Geometry: final body of the model. Coordinates: model frame, mm. A direction names the side the tool comes from. Round coordinates to 2 decimals unless told otherwise and drop trailing zeros. Loops run counter-clockwise (first coordinate to the right, second up) from the corner with the lowest first, then second, coordinate; pieces in that order, holes last. Notation, with made-up numbers: (-29.5, -0.75) - (-8.5, -0.75) arc R17 ccw to (-8.5, 11.25) - close; hole circle Ø11 at (15, 38.5). An arc over 180 degrees is marked (long way). Write item = value, one per line. Start each with the question number.
Item 1: Section B-B (y = 7.75). Return loops of the section in (x, z), plus the area to 3 significant figures.
Item 2: Line query: line 1 (Z direction, x = -1.75, y = 3); line 2 (X direction, y = 3.75, z = 3.5); line 3 (X direction, y = 5.25, z = 48). Output: solid intervals per line, ascending. Write a range as from..to.
Item 3: Access query for faces 5 (the flat face through (0, 2, 2.54)), 6 (the flat face through (-3.13, 5.58, 25.04)). Directions: +Z, -Z, +X, -X, +Y, -Y. A direction counts if a zero-diameter tool reaches every point of the face in a straight line with its end or side. Return the directions, or none.
Item 4: Section A-A (z = 34). Return loops of the section in (x, y), plus the area to 3 significant figures.
Item 5: Draft query along Z for faces 1 (the cylindrical face through (-0.02, 7.19, 25.1)), 2 (the flat face through (0, 2, 48.26)), 3 (the flat face through (0, 4, 50.8)), 4 (the flat face through (-5.2, 0, 23.4)). Return one class per face: pulls with the +Z half, pulls with the -Z half, needs draft (parallel to the pull), parting line crosses it, or undercut.
Item 6: First-contact query: pin 1 (2 mm diameter, centred on y = 6.5, z = 19.5, fed in from +X); pin 2 (3 mm diameter, centred on y = 9, z = 5, fed in from -X); pin 3 (1 mm diameter, centred on x = -2.5, y = 5, fed in from -Z); pin 4 (1 mm diameter, centred on y = 3.5, z = 15, fed in from -X). Flat tips, straight axial feed; report the tip coordinate or a pass-through.
from build123d import *

# Parameters (mm, degrees)
F1_DEPTH = 50.8
F4_DEPTH = 45.72
F5_R     = 1.27


with BuildPart() as f1:
    # F0 (on Top) → F1 (new body)
    with BuildSketch(Plane.XY):
        Polygon((-6.35, 0), (0, 0), (0, 10.9985226281), align=None)
        Polygon((0, 10.9985226281), (0, 0), (6.35, 0), align=None)
    extrude(amount=F1_DEPTH)

    # F3 (on offset) → F4 (cut)
    with BuildSketch(Plane.XY.offset(48.26)):
        Polygon((0, 8.4585226281), (-4.1502954744, 1.27), (4.1502954744, 1.27), align=None)
        Polygon((4.1502954744, 1.27), (-4.1502954744, 1.27), (-4.8835303163, 0), (4.8835303163, 0), align=None)
    extrude(amount=-F4_DEPTH, mode=Mode.SUBTRACT)

    # F5
    f5_edges = [f1.edges().sort_by_distance(p)[0] for p in [
        (0, 8.458523, 25.4),
        (2.441765, 4.229261, 2.54),
        (-2.441765, 4.229261, 2.54),
        (-2.441765, 4.229261, 48.26),
        (2.441765, 4.229261, 48.26),
    ]]
    fillet(f5_edges, radius=F5_R)


solid = f1.part
Taken from the geometry:
q1.outline = (-1.88, 0) - (1.88, 0) - (1.88, 50.8) - (-1.88, 50.8) - close
q1.area = 191 mm^2
q2.line_1 = 0..2.54, 48.26..50.8
q2.line_2 = -4.18..-2.67, 2.67..4.18
q2.line_3 = -3.32..-1.28, 1.28..3.32
q3.face_5 = -Y
q3.face_6 = +Z, -Z, -X, +Y
q4.outline = (-6.35, 0) - (-4.88, 0) - (-1.1, 6.55) arc R1.27 cw to (1.1, 6.55) - (4.88, 0) - (6.35, 0) - (0, 11) - close
q4.area = 29.6 mm^2
q5.face_1 = undercut
q5.face_2 = undercut
q5.face_3 = pulls with the +Z half
q5.face_4 = needs draft
q6.pin_1 = 3.17
q6.pin_2 = -2.02
q6.pin_3 = 0
q6.pin_4 = -4.62
